from build123d import *

# Parameters (mm, degrees)
SKETCH1_R               = 25
BOSS_EXTRUDE1_DEPTH     = 25
BOSS_EXTRUDE2_START     = 75
SKETCH1_2_R             = 25
BOSS_EXTRUDE2_DEPTH     = 75
CUT_EXTRUDE1_DEPTH      = 83.915619759
CUT_EXTRUDE1_DEPTH_BACK = 83.915619759
SKETCH2_W               = 25
SKETCH2_H               = 30
CUT_EXTRUDE2_DEPTH      = 83.915619759
CUT_EXTRUDE2_DEPTH_BACK = 83.915619759
SKETCH5_W               = 30
SKETCH5_H               = 13
CUT_EXTRUDE3_DEPTH      = 83.915619759
CUT_EXTRUDE3_DEPTH_BACK = 83.915619759
SKETCH6_W               = 30
SKETCH6_H               = 10
CUT_EXTRUDE4_DEPTH      = 83.915619759
CUT_EXTRUDE4_DEPTH_BACK = 83.915619759
SKETCH8_W               = 30
SKETCH8_H               = 36


with BuildPart() as part:
    # Sketch1 → Boss-Extrude1 (new body)
    with BuildSketch(Plane(origin=(0, 0, 0), x_dir=(-1, 0, 0), z_dir=(0, 1, 0))):
        with Locations(Location((0, 0, 0), (0, 0, 90))):
            Circle(SKETCH1_R)
    extrude(amount=-BOSS_EXTRUDE1_DEPTH)

    # Sketch1_2 → Boss-Extrude2 (add)
    with BuildSketch(Plane(origin=(0, 0, 0), x_dir=(-1, 0, 0), z_dir=(0, 1, 0)).offset(BOSS_EXTRUDE2_START)):
        with Locations(Location((0, 0, 0), (0, 0, 90))):
            Circle(SKETCH1_2_R)
    extrude(amount=-BOSS_EXTRUDE2_DEPTH)

    # Sketch2 → Cut-Extrude1 (cut, two sides: drawn at the far end of the back side and taken through both)
    with BuildSketch(Plane.YZ.offset(-CUT_EXTRUDE1_DEPTH_BACK)):
        with Locations((-12.5, 0)):
            Rectangle(SKETCH2_W, SKETCH2_H)
    extrude(amount=CUT_EXTRUDE1_DEPTH + CUT_EXTRUDE1_DEPTH_BACK, mode=Mode.SUBTRACT)

    # Sketch5 → Cut-Extrude2 (cut, two sides: drawn at the far end of the back side and taken through both)
    with BuildSketch(Plane.YZ.offset(-CUT_EXTRUDE2_DEPTH_BACK)):
        with Locations((60, 18.5)):
            Rectangle(SKETCH5_W, SKETCH5_H)
        with Locations((60, -18.5)):
            Rectangle(SKETCH5_W, SKETCH5_H)
    extrude(amount=CUT_EXTRUDE2_DEPTH + CUT_EXTRUDE2_DEPTH_BACK, mode=Mode.SUBTRACT)

    # Sketch6 → Cut-Extrude3 (cut, two sides: drawn at the far end of the back side and taken through both)
    with BuildSketch(Plane(origin=(0, 0, 0), x_dir=(0, 1, 0), z_dir=(0, 0, 1)).offset(-CUT_EXTRUDE3_DEPTH_BACK)):
        with Locations((-10, 0)):
            Rectangle(SKETCH6_W, SKETCH6_H)
    extrude(amount=CUT_EXTRUDE3_DEPTH + CUT_EXTRUDE3_DEPTH_BACK, mode=Mode.SUBTRACT)

    # Sketch8 → Cut-Extrude4 (cut, two sides: drawn at the far end of the back side and taken through both)
    with BuildSketch(Plane(origin=(0, 0, 0), x_dir=(0, 1, 0), z_dir=(0, 0, 1)).offset(-CUT_EXTRUDE4_DEPTH_BACK)):
        with Locations((60, 0)):
            Rectangle(SKETCH8_W, SKETCH8_H)
    extrude(amount=CUT_EXTRUDE4_DEPTH + CUT_EXTRUDE4_DEPTH_BACK, mode=Mode.SUBTRACT)


solid = part.part
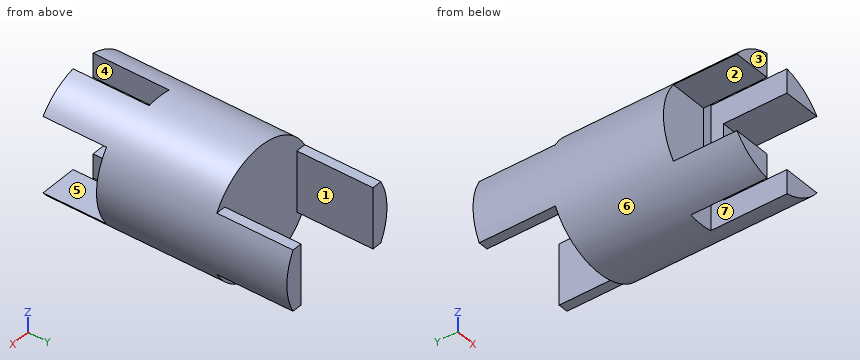
Model file for the job. Use its own axes, mm. Face numbers are marked on the shaded views. A direction names the side the tool comes from. Give positions to 0.01 mm unless a question says otherwise; leave off trailing zeros. Order: outer loops, then holes, each group sorted by start corner. A loop starts at its lowest first (then second) coordinate and runs counter-clockwise, first axis right, second up. Notation, with made-up numbers: M -23,41 L 23,41 A29 cw 23,73 Z; hole C 36,-4.75 d5. An arc over 180 degrees is marked long. Put each result on its own line as item: value. Start each with the question number.
(1) Drill centre lines: L1, parallel to X at y = 55, z = 0.5 (3 decimals); L2, parallel to Y at x = 8, z = -9.5; L3, parallel to Z at x = 0.5, y = 43.5 (3 decimals). Where is each one in solid material? Low to high. Write a range as [from, to].
(2) Tool access for the marked faces 1, 2, 3 and 4: list every direction of +Z, -Z, +X, -X, +Y, -Y with a clear straight run to the whole face (end or side of a thin tool).
(3) Band-saw the part on B-B on y = 53. Give the cut face in (x, z), then the cut area to 3 significant figures.
(4) Band-saw the part on D-D on x = 0. Give the cut face in (y, z).
(5) Pull direction Z, two halves, no side cores. Call the marked faces 5, 6 and 7: released by +Z, released by -Z, zero draft, split by the parting line, or undercut.
(6) Band-saw the part on C-C on z = 0. Give the cut face in (x, y).
(7) Pin check, flat tips, straight feed: pin 1 Ø12 at (y, z) = (62.5, 1.5) entering from +X; pin 2 Ø16.5 at (x, y) = (13.5, -9.5) entering from +Z; pin 3 Ø6 at (y, z) = (7, -8.5) entering from +X; pin 4 Ø16.5 at (x, y) = (10.5, -13.5) entering from -Z. Stop position of each tip, or through.
(8) Band-saw the part on A-A on y = -5. Give the cut face in (x, z), then the cut area to 3 significant figures.
Results below:
1. L1: x = [-24.995, -18], [18, 24.995]
1. L2: y = [0, 45]
1. L3: z = [-24.995, 24.995]
2. face 1: +Z, -Z, +Y
2. face 2: +X, -X, -Y
2. face 3: +Z, -Z, +X, -X, -Y
2. face 4: +Z, -Z, -Y
3. outline: M -21.93,-12 L -18,-12 L -18,12 L -21.93,12 A25 ccw Z; M 18,-12 L 21.93,-12 A25 ccw 21.93,12 L 18,12 Z
3. area: 288 mm2
4. outline: M 5,-25 L 45,-25 L 45,25 L 5,25 Z
5. face 5: undercut
5. face 6: split by the parting line
5. face 7: zero draft
6. outline: M -25,0 L -5,0 L -5,5 L 5,5 L 5,0 L 25,0 L 25,75 L 18,75 L 18,45 L -18,45 L -18,75 L -25,75 Z
7. pin 1: stops at x = 25
7. pin 2: stops at z = 24.44
7. pin 3: stops at x = 24.39
7. pin 4: stops at z = -24.49
8. outline: M -20,-15 A25 ccw -5,-24.49 L -5,-15 Z; M -20,15 L -5,15 L -5,24.49 A25 ccw Z; M 5,-24.49 A25 ccw 20,-15 L 5,-15 Z; M 5,15 L 20,15 A25 ccw 5,24.49 Z
8. area: 362 mm2
